The listing builds one solid part. Answer for the finished solid, in the listing's coordinates (mm). A direction names the side the tool comes from. Coordinates: 2 decimals unless noted, no trailing zeros. Order: outer loops, then holes, each group sorted by start corner. A loop starts at its lowest first (then second) coordinate and runs counter-clockwise, first axis right, second up. Notation, with made-up numbers: (47, 13) - (96, 13) arc R13 ccw to (96, 31) - close; hole circle Ø1 at (-4.5, -4). An arc over 180 degrees is marked (long way). Use a Markdown table: item, result. Add a question column.
Item 1: Find the intervals of material crossed by line 1 along Y through (x, z) = (-106.5, 2.7); line 2 along Y through (x, z) = (-107, 0.6); line 3 along Y through (x, z) = (-21, 0.65), in increasing order.
Item 2: For faces 5 (the flat face through (-64, 50.8, 2)), 6 (the flat face through (-19, -12.7, 2)), determine the directions among +Z, -Z, +X, -X, +Y, -Y from which every point of the face is accessible in a straight line to the end or side of a thin tool.
Item 3: The part is cut by section B-B, the plane y = 0. Give the vertices of the cut face in (x, z) (3 decimals).
Item 4: The part is cut by section C-C, the plane z = 0.5. State how many separate pieces and enclosed holes the cut face has, then the cut area to 3 significant figures.
Item 5: The part is cut by section D-D, the plane y = -21. Give the vertices of the cut face in (x, z) (3 decimals), then the cut area to 3 significant figures.
Item 6: The part is cut by section A-A, the plane y = 31.75. Give the vertices of the cut face in (x, z) (3 decimals).
Item 7: The mould has two halves that part along X. Classify faces 1 (the flat face through (-64, -1, 0)), 2 (the cylindrical face through (-64.646, 4.645, 1.565)), 3 (the flat face through (0, 19, 2)), 4 (the cylindrical face through (-39.543, -4.513, 1.565)): released by +X, released by -X, zero draft, split by the parting line, or undercut.
Item 8: A flat-ended cylindrical pin translates along its axis: P1, Ø4.5, axis at x = -40.894, y = -4.572, coming from the -Z side. Find the tip coordinate at first contact, or state that the pin passes through.
from build123d import *

# Parameters (mm, degrees)
F0_W            = 127
F0_H            = 3.175
F1_DEPTH        = 50.8
F3_D            = 3.3
F4_W            = 38.1
F4_H            = 38.1
F5_DEPTH        = 3.176
F7_D            = 2.2606
F10_D           = 2.2606
F12_D           = 2.7051
F14_D           = 4.9784
F14_CSINK_D     = 9.1186
F14_CSINK_ANGLE = 82


with BuildPart() as f1:
    # F0 (on Front) → F1 (new body, symmetric)
    with BuildSketch(Plane.XZ):
        with Locations((-63.5, 1.5875)):
            Rectangle(F0_W, F0_H)
    extrude(amount=F1_DEPTH, both=True)

    # F3 (through all)
    with Locations(Plane.XY.offset(3.175)):
        with Locations((-66.294, 4.572), (-66.294, -4.572), (-76.454, 0), (-96.52, 0), (-106.68, 4.572), (-106.68, -4.572)):
            Hole(F3_D / 2)

    # F4 (on face) → F5 (cut, through all)
    with BuildSketch(Plane.XY.offset(3.175)):
        with Locations((-19.05, -31.75)):
            Rectangle(F4_W, F4_H)
    extrude(amount=-F5_DEPTH, mode=Mode.SUBTRACT)

    # F7 (through all)
    with Locations(Plane.XY.offset(3.175)):
        with Locations((-4.7625, 19.05), (-26.9875, 19.05), (-26.9875, 44.45), (-4.7625, 44.45)):
            Hole(F7_D / 2)

    # F10 (through all)
    with Locations(Plane.XY.offset(3.175)):
        with Locations((-74.1045, -46.482), (-98.8695, -46.482), (-98.8695, -9.398), (-74.1045, -9.398)):
            Hole(F10_D / 2)

    # F12 (through all)
    with Locations(Plane.XY.offset(3.175)):
        with Locations((-40.894, -4.572), (-86.614, 3.81), (-86.614, 23.81)):
            Hole(F12_D / 2)

    # F14 (through all)
    with Locations(Plane(origin=(0, 0, 0), x_dir=(1, 0, 0), z_dir=(0, 0, -1))):
        with Locations((-30.1625, -31.75)):
            CounterSinkHole(F14_D / 2, F14_CSINK_D / 2, counter_sink_angle=F14_CSINK_ANGLE)


solid = f1.part
Solution:
| question | item | result |
|---|---|---|
| 1 | line 1 | y = -50.8 to -6.21, -2.93 to 2.93, 6.21 to 50.8 |
| 1 | line 2 | y = -50.8 to -6.19, -2.95 to 2.95, 6.19 to 50.8 |
| 1 | line 3 | y = -12.7 to 50.8 |
| 2 | face 5 | +Z, -Z, +X, -X, +Y |
| 2 | face 6 | +Z, -Z, +X, -Y |
| 3 | outline | (-127, 0) - (-98.17, 0) - (-98.17, 3.175) - (-127, 3.175) - close; (-94.87, 0) - (-78.104, 0) - (-78.104, 3.175) - (-94.87, 3.175) - close; (-74.804, 0) - (0, 0) - (0, 3.175) - (-74.804, 3.175) - close |
| 4 | separate pieces | 1 |
| 4 | enclosed holes | 18 |
| 4 | area | 11,300 mm2 |
| 5 | outline | (-127, 0) - (-38.1, 0) - (-38.1, 3.175) - (-127, 3.175) - close |
| 5 | area | 282 mm2 |
| 6 | outline | (-127, 0) - (-34.722, 0) - (-32.652, 2.381) - (-32.652, 3.175) - (-127, 3.175) - close; (-27.673, 2.381) - (-25.603, 0) - (0, 0) - (0, 3.175) - (-27.673, 3.175) - close |
| 7 | face 1 | zero draft |
| 7 | face 2 | undercut |
| 7 | face 3 | released by +X |
| 7 | face 4 | undercut |
| 8 | P1 | stops at z = 0 |
